```python
from build123d import *

# Parameters (mm, degrees)
SKETCH3_W           = 76
SKETCH3_H           = 8
SKETCH3_R           = 1.5
BOSS_EXTRUDE1_DEPTH = 5
SKETCH4_R           = 3
CUT_EXTRUDE1_DEPTH  = 3
SKETCH5_R           = 2.5
CUT_EXTRUDE2_DEPTH  = 3


with BuildPart() as part:
    # Sketch3 → Boss-Extrude1 (new body)
    with BuildSketch(Plane.XY.offset(4.5)):
        Rectangle(SKETCH3_W, SKETCH3_H)
        with Locations((-34.5, 0)):
            Circle(SKETCH3_R, mode=Mode.SUBTRACT)
        with Locations(Location((34.5, 0, 0), (0, 0, 180))):
            Circle(SKETCH3_R, mode=Mode.SUBTRACT)
    extrude(amount=BOSS_EXTRUDE1_DEPTH)

    # Sketch4 → Cut-Extrude1 (cut)
    with BuildSketch(Plane(origin=(0, 0, 4.5), x_dir=(-1, 0, 0), z_dir=(0, 0, -1))):
        Circle(SKETCH4_R)
    extrude(amount=-CUT_EXTRUDE1_DEPTH, mode=Mode.SUBTRACT)

    # Sketch5 → Cut-Extrude2 (cut)
    with BuildSketch(Plane.XY.offset(9.5)):
        with Locations((34.5, 0)):
            Circle(SKETCH5_R)
        with Locations(Location((-34.5, 0, 0), (0, 0, 180))):
            Circle(SKETCH5_R)
    extrude(amount=-CUT_EXTRUDE2_DEPTH, mode=Mode.SUBTRACT)


solid = part.part
```
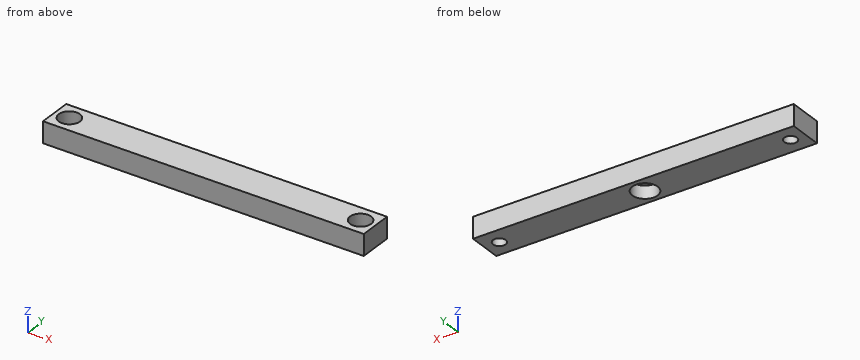
The model under review builds one solid part; all positions refer to its coordinate system, in mm. Round coordinates to 2 decimals unless told otherwise and drop trailing zeros. Loops run counter-clockwise (first coordinate to the right, second up) from the corner with the lowest first, then second, coordinate; pieces in that order, holes last. Notation, with made-up numbers: M -23.5,61 L 27.5,61 A34 ccw 27.5,97 Z; hole C 8,-21 d5. An arc over 180 degrees is marked long. Write item = value, one per line.
Item 1: For line 1 (X direction, y = -0.75, z = 6.8); line 2 (Y direction, x = 0, z = 5.8); line 3 (X direction, y = -1.5, z = 6.55), list the stretches that pass through material, from the lowest coordinate up. Write a range as [from, to].
Return value:
line_1 = [-38, -36.88], [-32.12, -2.9], [2.9, 32.12], [36.88, 38]
line_2 = [-4, -3], [3, 4]
line_3 = [-38, -36.5], [-32.5, -2.6], [2.6, 32.5], [36.5, 38]
Item 2: Take a section at C-C on z = 8.5. Write out the cut boundary in (x, y), then the cut area to 3 significant figures.
Return value:
outline = M -38,-4 L 38,-4 L 38,4 L -38,4 Z; hole C -34.5,0 d5; hole C 34.5,0 d5
area = 569 mm2
Item 3: Take a section at B-B on y = 0. Write out the cut boundary in (x, z), then the cut area to 3 significant figures.
Return value:
outline = M -38,4.5 L -36,4.5 L -36,6.5 L -37,6.5 L -37,9.5 L -38,9.5 Z; M -33,4.5 L -3,4.5 L -3,7.5 L 3,7.5 L 3,4.5 L 33,4.5 L 33,6.5 L 32,6.5 L 32,9.5 L -32,9.5 L -32,6.5 L -33,6.5 Z; M 36,4.5 L 38,4.5 L 38,9.5 L 37,9.5 L 37,6.5 L 36,6.5 Z
area = 320 mm2
Item 4: Take a section at A-A on x = 34.5. Write out the cut boundary in (y, z).
Return value:
outline = M -4,4.5 L -1.5,4.5 L -1.5,6.5 L -2.5,6.5 L -2.5,9.5 L -4,9.5 Z; M 1.5,4.5 L 4,4.5 L 4,9.5 L 2.5,9.5 L 2.5,6.5 L 1.5,6.5 Z
Item 5: Take a section at D-D on x = 0. Write out the cut boundary in (y, z), then the cut area to 3 significant figures.
Return value:
outline = M -4,4.5 L -3,4.5 L -3,7.5 L 3,7.5 L 3,4.5 L 4,4.5 L 4,9.5 L -4,9.5 Z
area = 22.0 mm2
Item 6: Insertion check: P1, Ø3, axis at x = 1, y = -1, coming from the -Z side. The pin has a flat end and moves straight along its axis. Give the tip position at first contact, or say it passes through.
Return value:
P1 = 7.5
